```python
from build123d import *

# Parameters (mm, degrees)
F0_R     = 1.7
F0_R_2   = 1.725
F1_DEPTH = 15
F2_W     = 3.5
F2_H     = 10.2
F3_DEPTH = 10
F4_R     = 1.7
F5_DEPTH = 5
F6_R     = 2
F7_DEPTH = 25
F9_DEPTH = 3


with BuildPart() as f1:
    # F0 (on Front) → F1 (new body)
    with BuildSketch(Plane.XZ):
        Polygon((-3.305435, 21.095744), (-3.305435, 31.295744), (-9.305435, 31.295744), (-11.805435, 28.695744), (-11.805435, 23.695744), (-9.305435, 21.095744), align=None)
        with Locations((-9.305435, 26.195744)):
            Circle(F0_R, mode=Mode.SUBTRACT)
        Polygon((1.194565, 33.795744), (-1.305435, 33.795744), (-3.305435, 31.795744), (-3.305435, 31.295744), (-3.305435, 21.095744), (-3.305435, 20.595744), (-1.305435, 18.595744), (1.194565, 18.595744), (3.194565, 20.595744), (3.194565, 31.795744), align=None)
        with Locations((-0.055435, 21.895744)):
            Circle(F0_R_2, mode=Mode.SUBTRACT)
        with Locations((-0.055435, 26.195744)):
            Circle(F0_R_2, mode=Mode.SUBTRACT)
        with Locations((-0.055435, 30.495744)):
            Circle(F0_R_2, mode=Mode.SUBTRACT)
    extrude(amount=F1_DEPTH)

    # F2 (on face) → F3 (join)
    with BuildSketch(Plane.XZ.offset(15)):
        with Locations((-5.055435, 26.195744)):
            Rectangle(F2_W, F2_H)
    extrude(amount=F3_DEPTH)

    # F4 (on face) → F5 (cut)
    with BuildSketch(Plane.XZ.offset(15)):
        Polygon((-6.805435, 21.095744), (-6.805435, 31.295744), (-9.305435, 31.295744), (-11.805435, 28.695744), (-11.805435, 23.695744), (-9.305435, 21.095744), align=None)
        with Locations((-9.305435, 26.195744)):
            Circle(F4_R, mode=Mode.SUBTRACT)
    extrude(amount=-F5_DEPTH, mode=Mode.SUBTRACT)

    # F6 (on face) → F7 (cut)
    with BuildSketch(Plane.YZ.offset(-3.305435)):
        with Locations((-20, 26.195744)):
            Circle(F6_R)
    extrude(amount=-F7_DEPTH, mode=Mode.SUBTRACT)

    # F8 (on face) → F9 (cut)
    with BuildSketch(Plane(origin=(0, 0, 0), x_dir=(-1, 0, 0), z_dir=(0, 1, 0))):
        with BuildLine():
            Line((11.084282, 29.445744), (9.305435, 29.445744))
            ThreePointArc((9.305435, 29.445744), (6.055435, 26.195744), (9.305435, 22.945744))
            Line((9.305435, 22.945744), (11.084282, 22.945744))
            Line((11.084282, 22.945744), (11.805435, 23.695744))
            Line((11.805435, 23.695744), (11.805435, 28.695744))
            Line((11.805435, 28.695744), (11.084282, 29.445744))
        make_face()
    extrude(amount=-F9_DEPTH, mode=Mode.SUBTRACT)


solid = f1.part
```
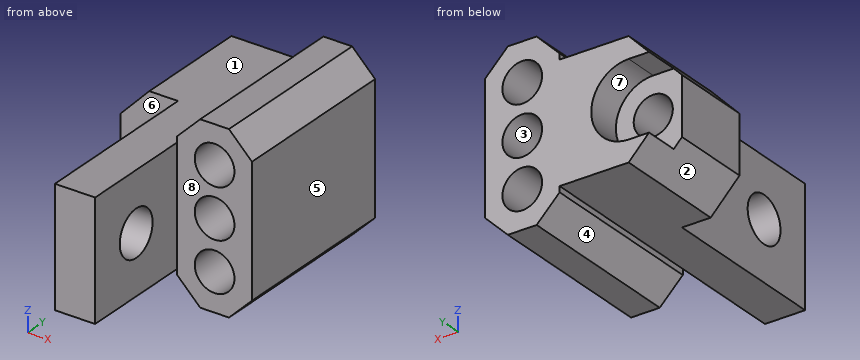
Work out the finished part from the listing and answer in its coordinate system (mm). Face numbers are marked on the shaded views. A direction names the side the tool comes from. Round coordinates to 2 decimals unless told otherwise and drop trailing zeros. Write each loop counter-clockwise with the first axis right and the second up, starting at its lowest first coordinate (ties: lowest second). Pieces come first, ordered by that corner, then holes. Notation, with made-up numbers: (65.25, 28.25) -> (122.25, 28.25) arc R26 cw to (122.25, 61.25) -> close; hole circle Ø6 at (89.25, 69.25). An arc over 180 degrees is marked (long way). Write each question's results on one line, items separated by ' | '.
1) Consider line 1 along X through (y, z) = (-9, 26.25); line 2 along Z through (x, y) = (-1.5, -13.5); line 3 along X through (y, z) = (-18.75, 23.25). Determine where each line is inside the solid, lowest interval first. Write a range as [from, to].
Findings:
line 1: x = [-11.81, -11], [-7.61, -1.78], [1.67, 3.19] | line 2: z = [18.79, 20.95], [22.84, 25.25], [27.14, 29.55], [31.44, 33.6] | line 3: x = [-6.81, -3.31]
2) Which of the six approach directions +Z, -Z, +X, -X, +Y, -Y give full straight-line access (tool end or side, diameter ignored) to the marked faces 4, 5, 6, 7 and 8?
Findings:
face 4: -Z, -X, +Y, -Y | face 5: +Z, -Z, +X, +Y, -Y | face 6: +Z, -Z, -X, -Y | face 7: -X, +Y | face 8: +Z, -Z, +X, -Y
3) The part is cut by section C-C (z = 29.75). Write down the section's boundary in (x, y), and give its area (3 significant figures).
Findings:
outline: (-10.79, -10) -> (-6.81, -10) -> (-6.81, -25) -> (-3.31, -25) -> (-3.31, -15) -> (-1.61, -15) -> (-1.61, 0) -> (-10.79, 0) -> close; (1.5, -15) -> (3.19, -15) -> (3.19, 0) -> (1.5, 0) -> close | area: 178 mm²
4) Flat-ended cylindrical pins translate along their axes: pin 1 (6 mm diameter, centred on x = -2.5, y = -21.5, fed in from -Z); pin 2 (5 mm diameter, centred on y = -13.5, z = 30.5, fed in from -X); pin 3 (5 mm diameter, centred on x = -2, y = -6.5, fed in from -Z); pin 4 (2.5 mm diameter, centred on x = -9, z = 28.5, fed in from -Y). Find the tip coordinate at first contact, or state that the pin passes through.
Findings:
pin 1: stops at z = 21.1 | pin 2: stops at x = -6.81 | pin 3: stops at z = 18.6 | pin 4: stops at y = -10
5) The part is cut by section D-D (y = -9.5). Write down the section's boundary in (x, z) (3 decimals), and give its area (3 significant figures).
Findings:
outline: (-11.805, 23.696) -> (-9.305, 21.096) -> (-3.305, 21.096) -> (-3.305, 20.596) -> (-1.305, 18.596) -> (1.195, 18.596) -> (3.195, 20.596) -> (3.195, 31.796) -> (1.195, 33.796) -> (-1.305, 33.796) -> (-3.305, 31.796) -> (-3.305, 31.296) -> (-9.305, 31.296) -> (-11.805, 28.696) -> close; hole circle Ø3.4 at (-9.305, 26.196); hole circle Ø3.45 at (-0.055, 21.896); hole circle Ø3.45 at (-0.055, 26.196); hole circle Ø3.45 at (-0.055, 30.496) | area: 134 mm²
6) For a pull along Z with two mould halves and no side action, classify the marked faces 1, 2 and 3 as +Z half, -Z half, draft (parallel to the pull), parting line (faces both ways), or undercut.
Findings:
face 1: +Z half | face 2: -Z half | face 3: undercut
7) The part is cut by section B-B (z = 27). Write down the section's boundary in (x, y).
Findings:
outline: (-11.81, -10) -> (-10.8, -10) -> (-10.8, -3) -> (-11.81, -3) -> close; (-7.81, -10) -> (-6.81, -10) -> (-6.81, -18.17) -> (-3.31, -18.17) -> (-3.31, -15) -> (-1.58, -15) -> (-1.58, 0) -> (-6.16, 0) -> (-6.16, -3) -> (-7.81, -3) -> close; (-6.81, -25) -> (-3.31, -25) -> (-3.31, -21.83) -> (-6.81, -21.83) -> close; (1.47, -15) -> (3.19, -15) -> (3.19, 0) -> (1.47, 0) -> close
8) The part is cut by section A-A (y = -20). Write down the section's boundary in (x, z).
Findings:
outline: (-6.81, 21.1) -> (-3.31, 21.1) -> (-3.31, 24.2) -> (-6.81, 24.2) -> close; (-6.81, 28.2) -> (-3.31, 28.2) -> (-3.31, 31.3) -> (-6.81, 31.3) -> close
